Here's how the part is built. I have some questions about the finished solid (model axes, mm). A direction names the side the tool comes from. Give positions to 0.01 mm unless a question says otherwise; leave off trailing zeros. Loops run counter-clockwise (first coordinate to the right, second up) from the corner with the lowest first, then second, coordinate; pieces in that order, holes last.
Q1. I need wall thicknesses on probe 1 along Y at (x, z) = (50, 2.9); probe 2 along X at (y, z) = (0.5, 0.45); probe 3 along X at (y, z) = (24, 3.7). Which ranges of each line are inside material? Lowest first, please.
Q2. I'm going to push flat-ended pins straight in: P1, Ø1.5, axis at x = 5.5, z = 3, coming from the +Y side; P2, Ø2.5, axis at x = 20.5, z = 2, coming from the +Y side. Where does each tip first touch, or does it pass through?
Q3. Suppose I cut it at A-A (z = 2). List the corners of the cut face in (x, y) for me.
Q4. Thinking about a two-plate mould opening in X: for faces 1 (the face through (10, 30, 2)), 2 (the face through (-10, 25, 2)), 3 (the face through (-0.325, 48.536, 2.465)), which applies, pulls with the +X half, pulls with the -X half, needs draft (parallel to the pull), parting line crosses it, or undercut?
Q5. Suppose I cut it at B-B (y = 12.5). List the corners of the cut face in (x, z) for me.
Q6. For faces 4 (the face through (0, 60, 2)), 5 (the face through (30, 10, 2)), which set-ups out of +Z, -Z, +X, -X, +Y, -Y let a thin tool reach every point of the face, with its end or its side?
```python
from build123d import *

# Parameters (mm, degrees)
SKETCH2_R           = 1.5
BOSS_EXTRUDE1_DEPTH = 5


with BuildPart() as part:
    # Sketch2 → Boss-Extrude1 (new body)
    with BuildSketch(Plane.XY):
        with BuildLine():
            Line((-10, 50), (-10, 0))
            ThreePointArc((-10, 0), (-7.071067812, -7.071067812), (0, -10))
            Line((0, -10), (50, -10))
            ThreePointArc((50, -10), (60, 0), (50, 10))
            Line((50, 10), (10, 10))
            Line((10, 10), (10, 50))
            ThreePointArc((10, 50), (0, 60), (-10, 50))
        make_face()
        Circle(SKETCH2_R, mode=Mode.SUBTRACT)
        with Locations((0, 50)):
            Circle(SKETCH2_R, mode=Mode.SUBTRACT)
        with Locations((50, 0)):
            Circle(SKETCH2_R, mode=Mode.SUBTRACT)
    extrude(amount=BOSS_EXTRUDE1_DEPTH)


solid = part.part
```
Solutions:
1. probe 1: y = -10 to -1.5, 1.5 to 10
1. probe 2: x = -10 to -1.41, 1.41 to 48.59, 51.41 to 59.99
1. probe 3: x = -10 to 10
2. P1: stops at y = 58.8
2. P2: stops at y = 10
3. outline: (-10, 0) arc R10 ccw to (0, -10) - (50, -10) arc R10 ccw to (50, 10) - (10, 10) - (10, 50) arc R10 ccw to (-10, 50) - close; hole circle Ø3 at (0, 0); hole circle Ø3 at (0, 50); hole circle Ø3 at (50, 0)
4. face 1: pulls with the +X half
4. face 2: pulls with the -X half
4. face 3: undercut
5. outline: (-10, 0) - (10, 0) - (10, 5) - (-10, 5) - close
6. face 4: +Z, -Z, +Y
6. face 5: +Z, -Z, +X, +Y
